Verification items for the finished model (mm, model axes). Face numbers are marked on the shaded views. A direction names the side the tool comes from. Give positions to 0.01 mm unless a question says otherwise; leave off trailing zeros. Order: outer loops, then holes, each group sorted by start corner. A loop starts at its lowest first (then second) coordinate and runs counter-clockwise, first axis right, second up. Notation, with made-up numbers: M -27.75,26.5 L -6.75,26.5 A25 ccw -6.75,55.5 Z; hole C -31.5,8.5 d9. An arc over 180 degrees is marked long. Answer as a JSON object with one key per item and string values.
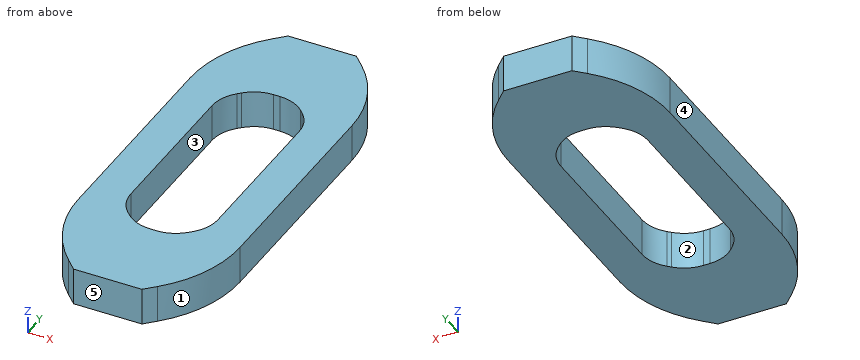
```python
from build123d import *

# Parameters (mm, degrees)
F1_DEPTH = 3
F2_R     = 3
F3_R     = 10


with BuildPart() as f1:
    # F0 (on Top) → F1 (new body)
    with BuildSketch(Plane.XY):
        Polygon((-6.5, 12.742641), (-6.5, 8.742641), (-6.5, -8.742641), (-6.5, -12.742641), (-2.742641, -16.5), (0, -16.5), (2.742641, -16.5), (6.5, -12.742641), (6.5, -8.742641), (6.5, 8.742641), (6.5, 12.742641), (2.742641, 16.5), (0, 16.5), (-2.742641, 16.5), align=None)
        Polygon((-3.5, 7.5), (-1.5, 9.5), (1.5, 9.5), (3.5, 7.5), (3.5, -7.5), (1.5, -9.5), (-1.5, -9.5), (-3.5, -7.5), align=None, mode=Mode.SUBTRACT)
    extrude(amount=F1_DEPTH)

    # F2
    f2_edges = [f1.edges().sort_by_distance(p)[0] for p in [
        (-3.5, 7.5, 1.5),
        (3.5, 7.5, 1.5),
        (3.5, -7.5, 1.5),
        (-3.5, -7.5, 1.5),
        (-1.5, 9.5, 1.5),
        (1.5, 9.5, 1.5),
        (1.5, -9.5, 1.5),
        (-1.5, -9.5, 1.5),
    ]]
    fillet(f2_edges, radius=F2_R)

    # F3
    f3_edges = [f1.edges().sort_by_distance(p)[0] for p in [
        (-6.5, 12.742641, 1.5),
        (6.5, 12.742641, 1.5),
        (6.5, -12.742641, 1.5),
        (-6.5, -12.742641, 1.5),
    ]]
    fillet(f3_edges, radius=F3_R)


solid = f1.part
```
Q1. Section check A-A on y = 2. Record the cut outline in (x, z).
Resolved:
{"outline": "M -6.5,0 L -3.5,0 L -3.5,3 L -6.5,3 Z; M 3.5,0 L 6.5,0 L 6.5,3 L 3.5,3 Z"}
Q2. Release check for a two-part mould opening along X. For the marked faces 3, 4 and 5 record: +X half, -X half, draft (parallel to the pull), parting line (faces both ways), or undercut.
Resolved:
{"face 3": "undercut", "face 4": "-X half", "face 5": "draft"}
Q3. Material ranges on L1, parallel to X at y = 4.5, z = 0.2; L2, parallel to Y at x = 0.25, z = 2.4; L3, parallel to Y at x = -1.25, z = 0.6, recorded low to high.
Resolved:
{"L1": "x = -6.5 to -3.5, 3.5 to 6.5", "L2": "y = -16.5 to -9.5, 9.5 to 16.5", "L3": "y = -16.5 to -9.33, 9.33 to 16.5"}
Q4. Section check D-D on y = -13. Record the cut outline in (x, z).
Resolved:
{"outline": "M -5.48,0 L 5.48,0 L 5.48,3 L -5.48,3 Z"}
Q5. Gauge pin test, flat ends, axial feed: pin 1 Ø1.5 at (y, z) = (-13, 2.5) entering from +X; pin 2 Ø5 at (x, y) = (1, 13) entering from -Z; pin 3 Ø1 at (y, z) = (-10, 0.5) entering from +X. Record the tip position at first contact, or that the pin passes through.
Resolved:
{"pin 1": "stops at x = 5.81", "pin 2": "stops at z = 0", "pin 3": "stops at x = 6.46"}
Q6. Section check B-B on z = 1. Record the cut outline in (x, y), then the cut area to 3 significant figures.
Resolved:
{"outline": "M -6.5,-8.6 A10 ccw -3.57,-15.67 L -2.74,-16.5 L 2.74,-16.5 L 3.57,-15.67 A10 ccw 6.5,-8.6 L 6.5,8.6 A10 ccw 3.57,15.67 L 2.74,16.5 L -2.74,16.5 L -3.57,15.67 A10 ccw -6.5,8.6 Z; hole M -3.5,-6.26 A3 ccw -2.62,-8.38 L -2.38,-8.62 A3 ccw -0.26,-9.5 L 0.26,-9.5 A3 ccw 2.38,-8.62 L 2.62,-8.38 A3 ccw 3.5,-6.26 L 3.5,6.26 A3 ccw 2.62,8.38 L 2.38,8.62 A3 ccw 0.26,9.5 L -0.26,9.5 A3 ccw -2.38,8.62 L -2.62,8.38 A3 ccw -3.5,6.26 Z", "area": "269 mm²"}
Q7. Section check C-C on x = -1. Record the cut outline in (y, z).
Resolved:
{"outline": "M -16.5,0 L -9.41,0 L -9.41,3 L -16.5,3 Z; M 9.41,0 L 16.5,0 L 16.5,3 L 9.41,3 Z"}
Q8. Tool access check on the marked faces 1 and 2. Record the directions out of +Z, -Z, +X, -X, +Y, -Y that give a thin tool (end or side, any length) a straight path to the whole face; none if there is none.
Resolved:
{"face 1": "+Z, -Z, +X, -Y", "face 2": "+Z, -Z"}
